Autodesk Inventor part; units mm, degrees
ref_plane "YZ Plane" through (0, 0, 0) normal (1, 0, 0) x (0, 1, 0)
ref_plane "XZ Plane" through (0, 0, 0) normal (0, 1, 0) x (-1, 0, 0)
ref_plane "XY Plane" through (0, 0, 0) normal (0, 0, 1) x (1, 0, 0)
sketch "Эскиз1" plane through (0, 0, 0) normal (0, 0, 1) x (1, 0, 0)
  circle A0 centre (0, 0) radius 3.25
  circle A1 centre (0, 0) radius 4.5
  dimension "d0" = 6.5
  dimension "d1" = 9
extrude "Выдавливание1" add sketch "Эскиз1" along normal blind 5.25
sketch "Эскиз2" plane through (0, 0, 0) normal (0, 0, -1) x (-1, 0, 0)
  circle A0 centre (0, 0) radius 5.5
  dimension "d4" = 11
loft "Лофт1" add profiles "Эскиз2" section 2 edges at (-4.5, 0, 5.25)
sketch "Эскиз4" plane through (0, 0, 0) normal (0, 0, -1) x (-1, 0, 0)
  circle A0 centre (0, 0) radius 3.25
  dimension "d10" = 6.5
extrude "Выдавливание2" cut sketch "Эскиз4" against normal through all
sketch "Эскиз5" plane through (0, 0, 0) normal (0, 0, -1) x (-1, 0, 0)
  circle A0 centre (-8.8669, 1.5421) radius 2.1
  circle A1 centre (-1.5421, -8.8669) radius 2.1
  circle A2 centre (1.5421, 8.8669) radius 2.1
  circle A3 centre (8.8669, -1.5421) radius 2.1
  circle A4 centre (0, 0) radius 13.5
  circle A5 centre (0, 0) radius 3.25
  dimension "d13" = 27
extrude "Выдавливание3" add sketch "Эскиз5" against normal blind 3
fillet "Сопряжение1" radius 2 1 edges at (4.9286, 0, 3)
chamfer "Фаска1" distance 2 angle 45 4 edges at (0.5579, 8.8669, 3) (10.9669, 1.5421, 3) (-6.7669, -1.5421, 3) (3.6421, -8.8669, 3)
sketch "Эскиз6" plane through (0, 0, 0) normal (0, 0, -1) x (-1, 0, 0)
  circle A0 centre (0, 0) radius 13.5
  circle A1 centre (8.8669, -1.5421) radius 2.1
  circle A2 centre (1.5421, 8.8669) radius 2.1
  circle A3 centre (-1.5421, -8.8669) radius 2.1
  circle A4 centre (-8.8669, 1.5421) radius 2.1
  circle A5 centre (0, 0) radius 3.25
extrude "Выдавливание4" cut sketch "Эскиз6" against normal blind 1
properties part number "втулка для крепл 2" material "Пластик ПЭТ"
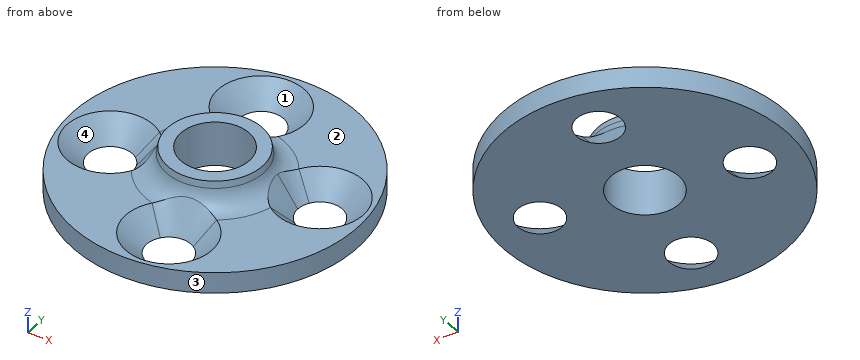
Can you work these out from the model? Positions are in its coordinate system, mm. Face numbers are marked on the shaded views. Coordinates: 2 decimals unless noted, no trailing zeros. Use a Markdown table: item, result.
Item 1: We'd pull the mould along X, two halves only. Please class the marked faces 1, 2, 3 and 4: released by +X, released by -X, zero draft, split by the parting line, or undercut.
Numbers:
| item | result |
|---|---|
| face 1 | undercut |
| face 2 | zero draft |
| face 3 | split by the parting line |
| face 4 | undercut |
Item 2: I want a section at A-A on y = 2.25. Give the number of separate pieces and of enclosed holes in the cut face, and give its area (3 significant figures).
Numbers:
| item | result |
|---|---|
| separate pieces | 3 |
| enclosed holes | 0 |
| area | 40.7 mm2 |
Item 3: If I drill on probe 1 along Y at (x, z) = (2, 2.15); probe 2 along Y at (x, z) = (0, 2.6); probe 3 along Z at (x, y) = (7.75, -7.75), over which ranges is the centre line in solid material (lowest first)? Write a range as from..to.
Numbers:
| item | result |
|---|---|
| probe 1 | y = -13.35..-12.08, -5.89..-2.56, 2.56..13.35 |
| probe 2 | y = -13.5..-12.23, -5.89..-3.25, 3.25..5.89, 12.23..13.5 |
| probe 3 | z = 1..3 |
Item 4: Will these pins go through, and if not, where does the flat tip stop? pin 1 (1 mm diameter, centred on x = -3.5, z = 4.5, fed in from +Y); pin 2 (13.5 mm diameter, centred on x = 2, y = 5, fed in from +Z); pin 3 (2 mm diameter, centred on y = -8.5, z = 3.5, fed in from +X).
Numbers:
| item | result |
|---|---|
| pin 1 | stops at y = 3.6 |
| pin 2 | stops at z = 5.25 |
| pin 3 | stops at x = 11.13 |
